The model under review builds one solid part; all positions refer to its coordinate system, in mm. Face numbers are marked on the shaded views. A direction names the side the tool comes from. Round coordinates to 2 decimals unless told otherwise and drop trailing zeros. Order: outer loops, then holes, each group sorted by start corner. A loop starts at its lowest first (then second) coordinate and runs counter-clockwise, first axis right, second up. Notation, with made-up numbers: (-14.5, -21) - (39.5, -21) arc R19 ccw to (39.5, -5) - close; hole circle Ø2 at (7, 74.5). An arc over 180 degrees is marked (long way). One line per question, with ' | ' between items. Start each with the question number.
Item 1: For L1, parallel to X at y = 33, z = 2.1; L2, parallel to X at y = 47, z = 0.9; L3, parallel to Y at x = 17.5, z = 1.15, list the stretches that pass through material, from the lowest coordinate up. Write a range as [from, to].
Item 2: Tool access review of the marked faces 1 and 2: name each direction out of +Z, -Z, +X, -X, +Y, -Y from which nothing blocks a thin tool from reaching the whole face with its end or side.
Item 3: Add section C-C on x = 19. State the section outline as (y, z) points (3 decimals).
Item 4: Add section D-D on y = 15. State the section outline as (x, z) points (3 decimals), and give its area (3 significant figures).
Item 5: Add section B-B on z = 2.35. State the section outline as (x, y) points, and give its area (3 significant figures).
Item 6: Draft analysis for pull direction Y (two halves, no side actions). For the marked faces 3, 4 and 5, state which applies: +Y half, -Y half, draft (parallel to the pull), parting line (faces both ways), or undercut.
Item 7: Insertion check: pin 1 Ø1.6 at (x, z) = (35.5, 1.5) entering from +Y; pin 2 Ø1.5 at (y, z) = (38, 1) entering from +X; pin 3 Ø1.6 at (y, z) = (29.5, 1.5) entering from -X. Each pin has a flat end and moves straight along its axis. Give the tip position at first contact, or say it passes through.
Item 8: Add section A-A on y = 42.5. State the section outline as (x, z) points (3 decimals), and give its area (3 significant figures).
from build123d import *

# Parameters (mm, degrees)
F1_DEPTH = 3.175
F2_R     = 5.08
F3_R     = 0.508


with BuildPart() as f1:
    # F0 (on Top) → F1 (new body)
    with BuildSketch(Plane.XY):
        Polygon((0, 12.7), (0, 0), (38.1, 0), (38.1, 12.7), (27.94, 12.7), (27.94, 45.72), (30.48, 45.72), (25.4, 50.8), (25.4, 12.7), (12.7, 12.7), (12.7, 50.8), (7.62, 45.72), (10.16, 45.72), (10.16, 12.7), align=None)
    extrude(amount=F1_DEPTH)

    # F2
    f2_edges = [f1.edges().sort_by_distance(p)[0] for p in [
        (27.94, 12.7, 1.5875),
        (25.4, 12.7, 1.5875),
        (12.7, 12.7, 1.5875),
        (10.16, 12.7, 1.5875),
    ]]
    fillet(f2_edges, radius=F2_R)

    # F3
    f3_edges = [f1.edges().sort_by_distance(p)[0] for p in [
        (27.94, 45.72, 1.5875),
        (30.48, 45.72, 1.5875),
        (10.16, 45.72, 1.5875),
        (7.62, 45.72, 1.5875),
        (12.7, 50.8, 1.5875),
        (25.4, 50.8, 1.5875),
    ]]
    fillet(f3_edges, radius=F3_R)


solid = f1.part
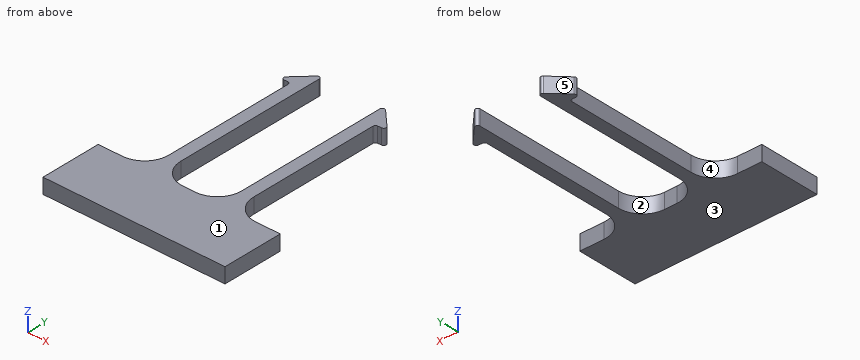
Determined:
1) L1: [10.16, 12.7], [25.4, 27.94] | L2: [8.9, 12.7], [25.4, 29.2] | L3: [0, 12.71]
2) face 1: +Z, +X, -X, +Y, -Y | face 2: +Z, -Z, +Y
3) outline: (0, 0) - (12.7, 0) - (12.7, 3.175) - (0, 3.175) - close
4) outline: (9.332, 0) - (13.528, 0) - (13.528, 3.175) - (9.332, 3.175) - close; (24.572, 0) - (28.768, 0) - (28.768, 3.175) - (24.572, 3.175) - close | area: 26.6 mm2
5) outline: (0, 0) - (38.1, 0) - (38.1, 12.7) - (33.02, 12.7) arc R5.08 cw to (27.94, 17.78) - (27.94, 45.21) arc R0.51 cw to (28.45, 45.72) - (29.25, 45.72) arc R0.51 ccw to (29.61, 46.59) - (26.27, 49.93) arc R0.51 ccw to (25.4, 49.57) - (25.4, 17.78) arc R5.08 cw to (20.32, 12.7) - (17.78, 12.7) arc R5.08 cw to (12.7, 17.78) - (12.7, 49.57) arc R0.51 ccw to (11.83, 49.93) - (8.49, 46.59) arc R0.51 ccw to (8.85, 45.72) - (9.65, 45.72) arc R0.51 cw to (10.16, 45.21) - (10.16, 17.78) arc R5.08 cw to (5.08, 12.7) - (0, 12.7) - close | area: 698 mm2
6) face 3: draft | face 4: undercut | face 5: +Y half
7) pin 1: y = 12.7 | pin 2: x = 27.94 | pin 3: x = 10.16
8) outline: (10.16, 0) - (12.7, 0) - (12.7, 3.175) - (10.16, 3.175) - close; (25.4, 0) - (27.94, 0) - (27.94, 3.175) - (25.4, 3.175) - close | area: 16.1 mm2
